```python
from build123d import *

# Parameters (mm, degrees)
SKETCH1_W           = 3.175
SKETCH1_H           = 254
BOSS_EXTRUDE1_DEPTH = 152.4
SKETCH2_W           = 79.375
SKETCH2_H           = 6.35
CUT_EXTRUDE1_DEPTH  = 3.175
SKETCH3_R           = 2.97688
CUT_EXTRUDE2_DEPTH  = 3.175


with BuildPart() as part:
    # Sketch1 → Boss-Extrude1 (new, symmetric)
    with BuildSketch(Plane(origin=(0, 0, 0), x_dir=(1, 0, 0), z_dir=(0, 1, 0))):
        Rectangle(SKETCH1_W, SKETCH1_H)
    extrude(amount=BOSS_EXTRUDE1_DEPTH, both=True)

    # Sketch2 → Cut-Extrude1 (cut)
    with BuildSketch(Plane(origin=(1.5875, 0, 0), x_dir=(0, 0, -1), z_dir=(1, 0, 0))):
        with Locations((0, -106.3625)):
            Rectangle(SKETCH2_W, SKETCH2_H)
    extrude(amount=-CUT_EXTRUDE1_DEPTH, mode=Mode.SUBTRACT)

    # Sketch3 → Cut-Extrude2 (cut)
    with BuildSketch(Plane(origin=(1.5875, 0, 0), x_dir=(0, 0, -1), z_dir=(1, 0, 0))):
        with Locations((117, 0)):
            Circle(SKETCH3_R)
        with Locations((117, 101.6)):
            Circle(SKETCH3_R)
        with Locations(Location((117, -101.6, 0), (0, 0, 180))):
            Circle(SKETCH3_R)
        with Locations((-117, -101.6)):
            Circle(SKETCH3_R)
        with Locations(Location((-117, 0, 0), (0, 0, 180))):
            Circle(SKETCH3_R)
        with Locations(Location((-117, 101.6, 0), (0, 0, 180))):
            Circle(SKETCH3_R)
    extrude(amount=-CUT_EXTRUDE2_DEPTH, mode=Mode.SUBTRACT)


solid = part.part
```
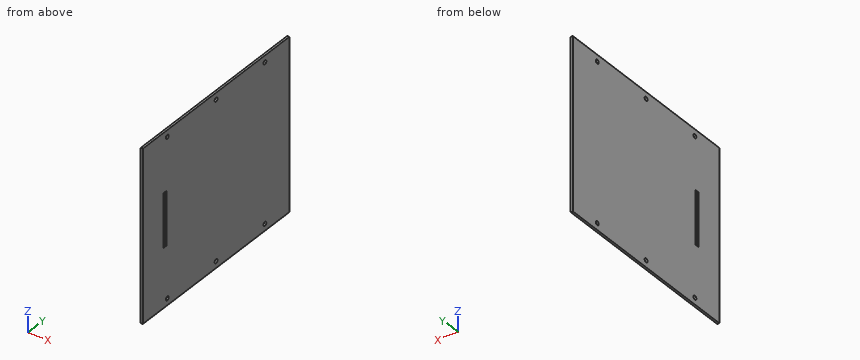
CAD build for the part. Positions are in the model's coordinates, mm. Round coordinates to 2 decimals unless told otherwise and drop trailing zeros. Loops run counter-clockwise (first coordinate to the right, second up) from the corner with the lowest first, then second, coordinate; pieces in that order, holes last. Notation, with made-up numbers: M -7,-18.75 L 29,-18.75 A11 cw 29,-4.75 Z; hole C -17,7.5 d8. An arc over 180 degrees is marked long. Use a Markdown table: item, result. Add a question column.
(1) Flat gauge pins, fed straight in: pin 1 (7 mm diameter, centred on y = 0, z = -117, fed in from +X); pin 2 (5.5 mm diameter, centred on y = -101.6, z = -117, fed in from -X). Where does each tip first touch, or does it go through?
(2) Cut at A-A (z = 11). Give the cut face in (x, y).
(3) Drill centre lines: line 1 (Y direction, x = 1.25, z = -116.5); line 2 (Y direction, x = -0.3, z = -117); line 3 (Z direction, x = -1.35, y = -108.5). Where is each one in solid material? Low to high.
Geometry says:
| question | item | result |
|---|---|---|
| 1 | pin 1 | stops at x = 1.59 |
| 1 | pin 2 | passes through |
| 2 | outline | M -1.59,-152.4 L 1.59,-152.4 L 1.59,-109.54 L -1.59,-109.54 Z; M -1.59,-103.19 L 1.59,-103.19 L 1.59,152.4 L -1.59,152.4 Z |
| 3 | line 1 | y = -152.4 to -104.53, -98.67 to -2.93, 2.93 to 98.67, 104.53 to 152.4 |
| 3 | line 2 | y = -152.4 to -104.58, -98.62 to -2.98, 2.98 to 98.62, 104.58 to 152.4 |
| 3 | line 3 | z = -127 to -39.69, 39.69 to 127 |
